Study the drawing (mm; zero at the part's minimum x, y, z) and answer. A direction names the side the tool comes from. Round coordinates to 2 decimals unless told otherwise and drop trailing zeros. Write each loop counter-clockwise with the first axis right and the second up, starting at its lowest first coordinate (ties: lowest second). Pieces come first, ordered by that corner, then holes. Notation, with made-up numbers: M 81.5,42 L 110.5,42 A14 cw 110.5,59 Z; hole C 55,81.25 d5. An arc over 180 degrees is marked long. Write each question's results on one line, items separated by ' | '.
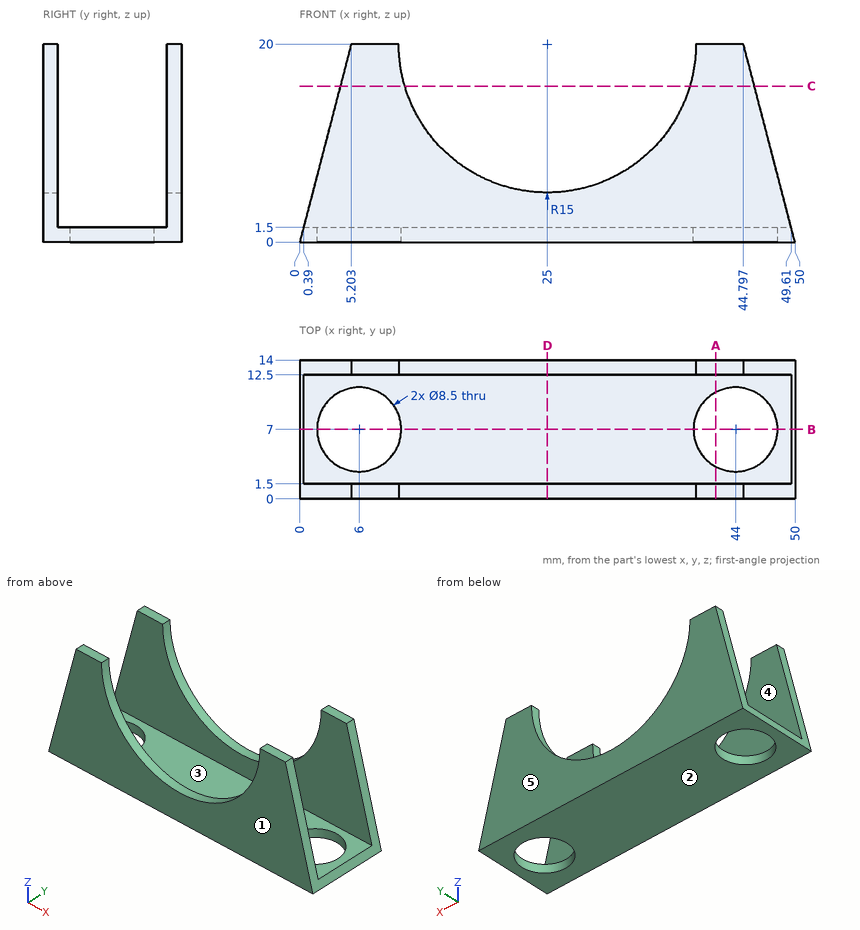
1) Each of these flat-tipped pins is pushed along its axis until it touches: pin 1 (5 mm diameter, centred on y = 12.5, z = 13, fed in from +X); pin 2 (3.5 mm diameter, centred on x = 18.5, y = 8, fed in from +Z). Where does it stop, or does it pass through?
Return value:
pin 1: x = 47.27 | pin 2: z = 1.5
2) Section A-A (x = 42) is taken. Determine the outline of the cut face in (y, z).
Return value:
outline: M 0,0 L 3.25,0 L 3.25,1.5 L 1.5,1.5 L 1.5,20 L 0,20 Z; M 10.75,0 L 14,0 L 14,20 L 12.5,20 L 12.5,1.5 L 10.75,1.5 Z
3) Section D-D (x = 25) is taken. Determine the outline of the cut face in (y, z).
Return value:
outline: M 0,0 L 14,0 L 14,5 L 12.5,5 L 12.5,1.5 L 1.5,1.5 L 1.5,5 L 0,5 Z
4) The mould has two halves that part along Y. Classify the marked faces 1, 2 and 3: +Y half, -Y half, draft (parallel to the pull), parting line (faces both ways), or undercut.
Return value:
face 1: -Y half | face 2: draft | face 3: undercut
5) A tool of negligible diameter and unlimited length cuts with its end or side. For the marked faces 4 and 5, from which of +Z, -Z, +X, -X, +Y, -Y can it reach the whole face along a straight path? Write none if from no direction.
Return value:
face 4: +Z, +X, -X | face 5: +Z, -Z, +X, -X, +Y
6) Find the intervals of material crossed by line 1 (Y direction, x = 6, z = 0.5); line 2 (Y direction, x = 43.5, z = 9.5); line 3 (Z direction, x = 48, y = 10), in increasing order.
Return value:
line 1: 0 to 2.75, 11.25 to 14 | line 2: 0 to 1.5, 12.5 to 14 | line 3: 0 to 1.5
7) Section B-B (y = 7) is taken. Determine the outline of the cut face in (x, z).
Return value:
outline: M 0,0 L 1.75,0 L 1.75,1.5 L 0.39,1.5 Z; M 10.25,0 L 39.75,0 L 39.75,1.5 L 10.25,1.5 Z; M 48.25,0 L 50,0 L 49.61,1.5 L 48.25,1.5 Z
8) Section C-C (z = 15.75) is taken. Determine the outline of the cut face in (x, y) (1 decimal).
Return value:
outline: M 4.1,0 L 10.6,0 L 10.6,1.5 L 4.1,1.5 Z; M 4.1,12.5 L 10.6,12.5 L 10.6,14 L 4.1,14 Z; M 39.4,0 L 45.9,0 L 45.9,1.5 L 39.4,1.5 Z; M 39.4,12.5 L 45.9,12.5 L 45.9,14 L 39.4,14 Z
